Design review of the part built by this model. Coordinates are the model's own, in mm. Coordinates: 2 decimals unless noted, no trailing zeros. Write each loop counter-clockwise with the first axis right and the second up, starting at its lowest first coordinate (ties: lowest second). Pieces come first, ordered by that corner, then holes. Notation, with made-up numbers: M 79,-5 L 107,-5 A24 ccw 107,5 Z; hole C 0,57 d9. An arc over 180 degrees is marked long. One line per question, with ' | ' between items.
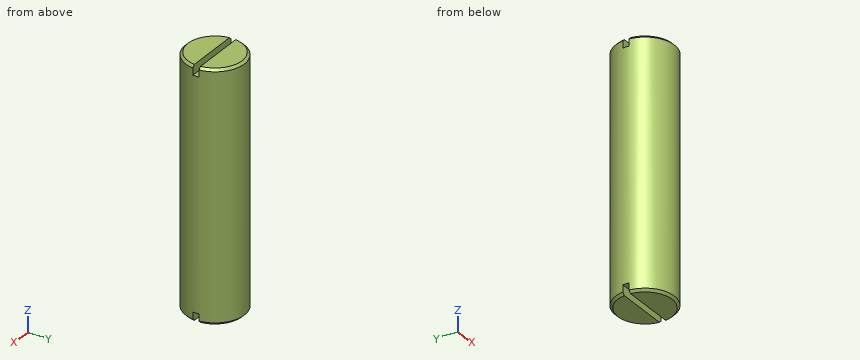
from build123d import *

# Parameters (mm, degrees)
SKETCH1_R               = 9.525
BOSS_EXTRUDE1_DEPTH     = 40
CHAMFER1_SIZE           = 0.762
SKETCH2_W               = 3
SKETCH2_H               = 2
CUT_EXTRUDE1_DEPTH      = 10.525
CUT_EXTRUDE1_DEPTH_BACK = 10.525


with BuildPart() as part:
    # Sketch1 → Boss-Extrude1 (new body, symmetric)
    with BuildSketch(Plane.XY):
        Circle(SKETCH1_R)
    extrude(amount=BOSS_EXTRUDE1_DEPTH, both=True)

    # Chamfer1
    chamfer1_edges = [part.edges().sort_by_distance(p)[0] for p in [
        (-9.525, 0, -40),
        (-9.525, 0, 40),
    ]]
    chamfer(chamfer1_edges, length=CHAMFER1_SIZE)

    # Sketch2 → Cut-Extrude1 (cut, two sides)
    with BuildSketch(Plane(origin=(0, 0, 0), x_dir=(0, 0, -1), z_dir=(1, 0, 0))) as cut_extrude1_sk:
        with Locations((-38.5, 0)):
            Rectangle(SKETCH2_W, SKETCH2_H)
        with Locations((38.5, 0)):
            Rectangle(SKETCH2_W, SKETCH2_H)
    extrude(amount=CUT_EXTRUDE1_DEPTH, mode=Mode.SUBTRACT)
    extrude(cut_extrude1_sk.sketch, amount=-CUT_EXTRUDE1_DEPTH_BACK, mode=Mode.SUBTRACT)


solid = part.part
1. Take a section at A-A (y = 0). Write out the cut boundary in (x, z) (3 decimals), then the cut area to 3 significant figures.
Answer sheet:
outline: M -9.525,-37 L 9.525,-37 L 9.525,37 L -9.525,37 Z | area: 1,410 mm^2
2. To check wall thickness, follow line 1 along Z through (x, y) = (-5, 0.25); line 2 along X through (y, z) = (3.75, -26.5); line 3 along Y through (x, z) = (0.5, -16.5). State the ranges of each line that lie inside material, in increasing order. Write a range as [from, to].
Answer sheet:
line 1: [-37, 37] | line 2: [-8.76, 8.76] | line 3: [-9.51, 9.51]
3. Insertion check: pin 1 Ø1.5 at (x, z) = (-4, 38.5) entering from +Y; pin 2 Ø1.5 at (x, z) = (-4.5, -38) entering from +Y; pin 3 Ø3.5 at (x, z) = (3, 39) entering from -Y. Each pin has a flat end and moves straight along its axis. Give the tip position at first contact, or say it passes through.
Answer sheet:
pin 1: y = 8.95 | pin 2: y = 8.76 | pin 3: y = -9.44
4. Take a section at B-B (z = 16). Write out the cut boundary in (x, y) (3 decimals).
Answer sheet:
outline: C 0,0 d19.05
